Source: three-view drawing plus pictorial views. Frame: mm from the lowest corner of the part. A direction names the side the tool comes from. Coordinates: 2 decimals unless noted, no trailing zeros. Loops run counter-clockwise (first coordinate to the right, second up) from the corner with the lowest first, then second, coordinate; pieces in that order, holes last.
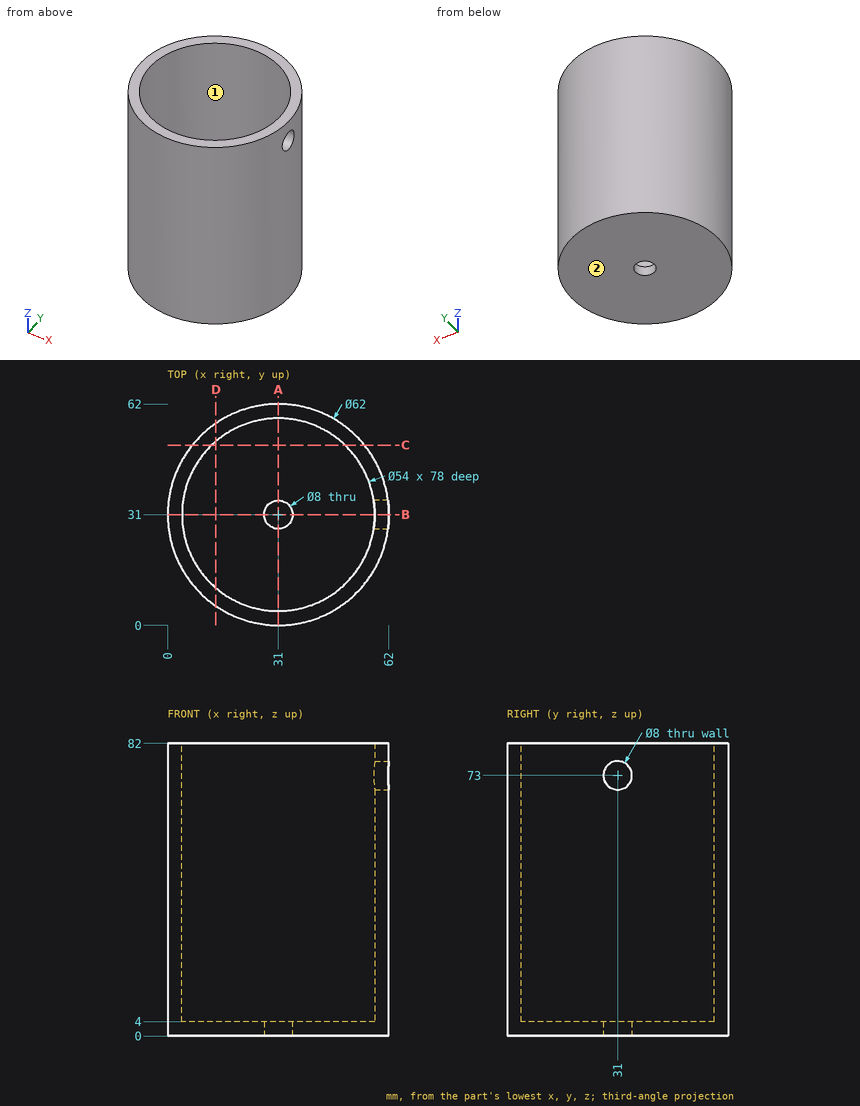
Q1. Section C-C, the plane y = 50.5. Return the cut outline in (x, z), plus the area to 3 significant figures.
Q2. Section B-B, the plane y = 31. Return the cut outline in (x, z), plus the area to 3 significant figures.
Q3. Line query: line 1 along Y through (x, z) = (31, 27); line 2 along Z through (x, y) = (20, 43.5). Output: solid intervals per line, ascending.
Q4. Section A-A, the plane x = 31. Return the cut outline in (y, z), plus the area to 3 significant figures.
Q5. Contact query for flat-ended pins moving along their axis: pin 1 Ø10 at (x, z) = (26, 73) entering from +Y; pin 2 Ø5 at (y, z) = (31, 73) entering from +X; pin 3 Ø5 at (x, y) = (44.5, 46) entering from +Z. Output: stop coordinate, or through.
Q6. Section D-D, the plane x = 13.5. Return the cut outline in (y, z).
Q7. Access query for the marked faces 1 and 2. Directions: +Z, -Z, +X, -X, +Y, -Y. A direction counts if a zero-diameter tool reaches every point of the face in a straight line with its end or side. Return the directions, or none.
Derived:
1. outline: (6.9, 0) - (55.1, 0) - (55.1, 82) - (49.67, 82) - (49.67, 4) - (12.33, 4) - (12.33, 82) - (6.9, 82) - close
1. area: 1,040 mm2
2. outline: (0, 0) - (27, 0) - (27, 4) - (4, 4) - (4, 82) - (0, 82) - close; (35, 0) - (62, 0) - (62, 69) - (58, 69) - (58, 4) - (35, 4) - close; (58, 77) - (62, 77) - (62, 82) - (58, 82) - close
2. area: 808 mm2
3. line 1: y = 0 to 4, 58 to 62
3. line 2: z = 0 to 4
4. outline: (0, 0) - (27, 0) - (27, 4) - (4, 4) - (4, 82) - (0, 82) - close; (35, 0) - (62, 0) - (62, 82) - (58, 82) - (58, 4) - (35, 4) - close
4. area: 840 mm2
5. pin 1: stops at y = 62
5. pin 2: stops at x = 4.12
5. pin 3: stops at z = 4
6. outline: (5.41, 0) - (56.59, 0) - (56.59, 82) - (51.56, 82) - (51.56, 4) - (10.44, 4) - (10.44, 82) - (5.41, 82) - close
7. face 1: +Z
7. face 2: -Z, +X, -X, +Y, -Y
